The model under review builds one solid part; all positions refer to its coordinate system, in mm. A direction names the side the tool comes from. Give positions to 0.01 mm unless a question says otherwise; leave off trailing zeros. Loops run counter-clockwise (first coordinate to the right, second up) from the corner with the lowest first, then second, coordinate; pieces in that order, holes last. Notation, with made-up numbers: M 8,54 L 48,54 A13 ccw 48,68 Z; hole C 27,1.25 d8. An arc over 180 degrees is marked long. Put each result on its own line as item: value. Start each with the question number.
from build123d import *

# Parameters (mm, degrees)
F0_W     = 29.2758359574
F0_H     = 5.0876662135
F0_W_2   = 5.8360383846
F0_H_2   = 27.9592750594
F1_DEPTH = 7.112


with BuildPart() as f1:
    # F0 (on Right) → F1 (new body)
    with BuildSketch(Plane.YZ):
        with Locations((-20.4739563633, 35.8995459974)):
            Rectangle(F0_W, F0_H)
        with Locations((-2.9180191923, 35.8995459974)):
            Rectangle(F0_W_2, F0_H)
        with Locations((-2.9180191923, 19.3760753609)):
            Rectangle(F0_W_2, F0_H_2)
    extrude(amount=F1_DEPTH)


solid = f1.part
(1) We need section A-A, the plane z = 16. Write out the cut boundary in (x, y).
(2) Insertion check: pin 1 (2 mm diameter, centred on x = 5, y = -16, fed in from -Z); pin 2 (2 mm diameter, centred on x = 2.5, z = 22, fed in from -Y). Each pin has a flat end and moves straight along its axis. Give the tip position at first contact, or say it passes through.
(3) We need section C-C, the plane y = -18.5. Write out the cut boundary in (x, z), plus the area to 3 significant figures.
(4) To check wall thickness, follow L1, parallel to Z at x = 6, y = -25; L2, parallel to Y at x = 1.5, z = 12.5. State the ranges of each line that lie inside material, in increasing order. Write a range as [from, to].
(5) We need section B-B, the plane x = 2. Write out the cut boundary in (y, z).
(6) For faces 1 (the flat face through (4, -35.112, 36)), 2 (the flat face through (4, -21, 33.356)), list the 3-axis set-ups (+Z, -Z, +X, -X, +Y, -Y) from which the entire face can be reached by the end or side of a thin tool; tool diameter is ignored.
Check sheet entries:
1. outline: M 0,-5.84 L 7.11,-5.84 L 7.11,0 L 0,0 Z
2. pin 1: stops at z = 33.36
2. pin 2: stops at y = -5.84
3. outline: M 0,33.36 L 7.11,33.36 L 7.11,38.44 L 0,38.44 Z
3. area: 36.2 mm²
4. L1: z = [33.36, 38.44]
4. L2: y = [-5.84, 0]
5. outline: M -35.11,33.36 L -5.84,33.36 L -5.84,5.4 L 0,5.4 L 0,38.44 L -35.11,38.44 Z
6. face 1: +Z, -Z, +X, -X, -Y
6. face 2: -Z, +X, -X, -Y
